Check sheet for the drawn part. Datum: minimum x, y, z corner. Units: mm. Coordinates: 2 decimals unless noted, no trailing zeros. Write each loop counter-clockwise with the first axis right and the second up, starting at its lowest first coordinate (ties: lowest second). Pieces come first, ordered by that corner, then holes. Notation, with made-up numbers: M 36,72 L 68,72 A24 ccw 68,88 Z; hole C 34.5,60 d4. An arc over 180 degrees is marked long. Answer as CSV lines item,"result".
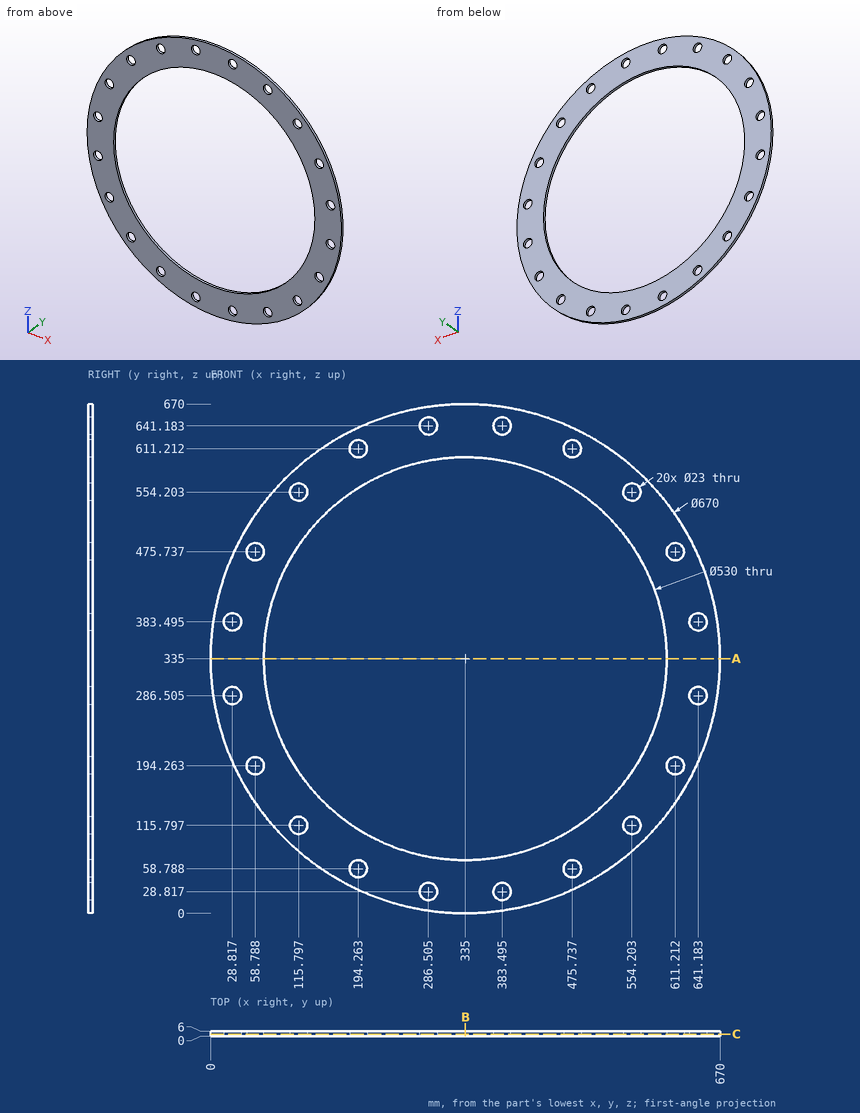
1) Section check C-C, the plane y = 2.5. Give the number of separate pieces and of enclosed holes in the cut face, plus the area to 3 significant figures.
Answer key:
separate pieces,"1"
enclosed holes,"21"
area,"124,000 mm2"
2) Thickness scan on line 1 along Z through (x, y) = (479, 4.1) (1 decimal); line 2 along X through (y, z) = (5.25, 30) (1 decimal); line 3 along X through (y, z) = (2.8, 335). Record the ranges inside material, lowest first.
Answer key:
line 1,"z = 32.5 to 47.8, 69.8 to 112.5, 557.5 to 600.2, 622.2 to 637.5"
line 2,"x = 196.4 to 275.1, 297.9 to 372.1, 394.9 to 473.6"
line 3,"x = 0 to 70, 600 to 670"
3) Section check B-B, the plane x = 335. Record the boundary of the cut face in (y, z), plus the area to 3 significant figures.
Answer key:
outline,"M 0,0 L 6,0 L 6,70 L 0,70 Z; M 0,600 L 6,600 L 6,670 L 0,670 Z"
area,"840 mm2"
4) Section check A-A, the plane z = 335. Record the boundary of the cut face in (x, y), plus the area to 3 significant figures.
Answer key:
outline,"M 0,0 L 70,0 L 70,6 L 0,6 Z; M 600,0 L 670,0 L 670,6 L 600,6 Z"
area,"840 mm2"
